from build123d import *

# Parameters (mm, degrees)
SKETCH_R             = 55
PAD_DEPTH            = 28
SKETCH001_R          = 52.5
PAD001_DEPTH         = 16
SKETCH012_R          = 50
PAD005_DEPTH         = 30
BODY_PLACEMENT_ANGLE = 90


with BuildPart() as part:
    # Sketch → Pad (new body)
    with BuildSketch(Plane.XY):
        with Locations((0.027552, 0)):
            Circle(SKETCH_R)
    extrude(amount=PAD_DEPTH)

    # Sketch001 (on Face3 of Pad) → Pad001 (join)
    with BuildSketch(Plane.XY.offset(28)):
        Circle(SKETCH001_R)
    extrude(amount=PAD001_DEPTH)

    # Sketch012 (on Face5 of Pad001) → Pad005 (join)
    with BuildSketch(Plane.XY.offset(44)):
        Circle(SKETCH012_R)
    extrude(amount=PAD005_DEPTH)


with BuildPart() as part_1:
    # Body placement: moved
    add(part.part.moved(Location((0, -23, 0))).rotate(Axis((0, -23, 0), (-1, 0, 0)), BODY_PLACEMENT_ANGLE))


solid = part_1.part
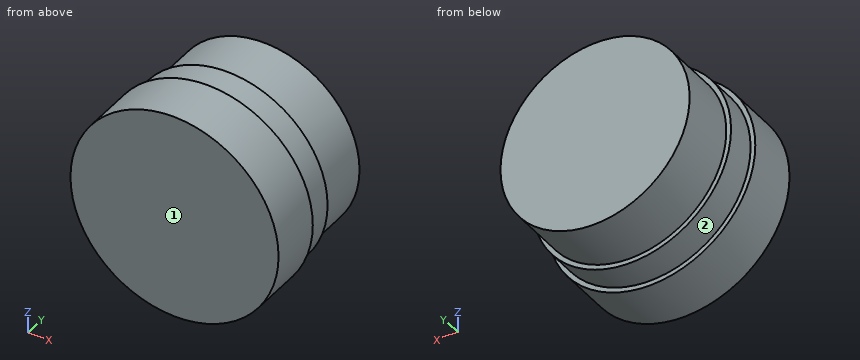
Geometry: final body of the model. Coordinates: model frame, mm. Face numbers are marked on the shaded views. A direction names the side the tool comes from. Round coordinates to 2 decimals unless told otherwise and drop trailing zeros. Loops run counter-clockwise (first coordinate to the right, second up) from the corner with the lowest first, then second, coordinate; pieces in that order, holes last.
Q1. Section A-A on z = 0. Return loops of the section in (x, y).
Q2. Material intervals for L1, parallel to Y at x = 8.5, z = -49.5; L2, parallel to Y at x = -46, z = 28.5; L3, parallel to Z at x = -32, y = 36, sorted ascending.
Q3. Section B-B on x = 0. Return loops of the section in (y, z).
Q4. Pin query (flat end, axial travel): P1, Ø3, axis at y = 17, z = -33.5, coming from the +X side; P2, Ø2, axis at y = 34, z = -40.5, coming from the +X side; P3, Ø4, axis at x = -32, y = -6, coming from the -Z side. Return the tip coordinate at first contact, or that it passes through.
Q5. Access query for the marked faces 1 and 2. Directions: +Z, -Z, +X, -X, +Y, -Y. A direction counts if a zero-diameter tool reaches every point of the face in a straight line with its end or side. Return the directions, or none.
Q6. Section D-D on y = 31. Return loops of the section in (x, z).
Q7. Section C-C on y = 1. Return loops of the section in (x, z).
Evaluation:
1. outline: (-54.97, -23) - (55.03, -23) - (55.03, 5) - (52.5, 5) - (52.5, 21) - (50, 21) - (50, 51) - (-50, 51) - (-50, 21) - (-52.5, 21) - (-52.5, 5) - (-54.97, 5) - close
2. L1: y = -23 to 21
2. L2: y = -23 to 5
2. L3: z = -38.42 to 38.42
3. outline: (-23, -55) - (5, -55) - (5, -52.5) - (21, -52.5) - (21, -50) - (51, -50) - (51, 50) - (21, 50) - (21, 52.5) - (5, 52.5) - (5, 55) - (-23, 55) - close
4. P1: stops at x = 41.62
4. P2: stops at x = 30.66
4. P3: stops at z = -46.08
5. face 1: +Z, -Z, +X, -X, -Y
5. face 2: +Y
6. outline: circle Ø100 at (0, 0)
7. outline: circle Ø110 at (0.03, 0)
